from build123d import *

# Parameters (mm, degrees)
F0_W     = 38.1
F0_H     = 76.2
F1_DEPTH = 12.7
F2_R     = 9.525
F3_DEPTH = 38.1
F4_R     = 6.35
F5_DEPTH = 40.386
F6_R     = 2.54
F7_DEPTH = 25.4
F8_R     = 4.445
F9_DEPTH = 7.62


with BuildPart() as f1:
    # F0 (on Front) → F1 (new body)
    with BuildSketch(Plane.XZ):
        Rectangle(F0_W, F0_H)
    extrude(amount=F1_DEPTH)

    # F2 (on face) → F3 (join)
    with BuildSketch(Plane.YZ.offset(19.05)):
        with Locations((-12.7, 0)):
            Circle(F2_R)
    extrude(amount=-F3_DEPTH)

    # F4 (on face) → F5 (cut)
    with BuildSketch(Plane.YZ.offset(19.05)):
        with Locations((-12.7, 0)):
            Circle(F4_R)
    extrude(amount=-F5_DEPTH, mode=Mode.SUBTRACT)

    # F6 (on face) → F7 (cut)
    with BuildSketch(Plane.XZ.offset(12.7)):
        with Locations((-7.62, 25.4)):
            Circle(F6_R)
        with Locations((7.62, 25.4)):
            Circle(F6_R)
        with Locations((-7.62, -25.4)):
            Circle(F6_R)
        with Locations((7.62, -25.4)):
            Circle(F6_R)
    extrude(amount=-F7_DEPTH, mode=Mode.SUBTRACT)

    # F8 (on face) → F9 (cut)
    with BuildSketch(Plane.XZ.offset(12.7)):
        with Locations((-7.62, 25.4)):
            Circle(F8_R)
        with Locations((7.62, 25.4)):
            Circle(F8_R)
        with Locations((-7.62, -25.4)):
            Circle(F8_R)
        with Locations((7.62, -25.4)):
            Circle(F8_R)
    extrude(amount=-F9_DEPTH, mode=Mode.SUBTRACT)


solid = f1.part
Design review of the part built by this model. Coordinates are the model's own, in mm. A direction names the side the tool comes from. Coordinates: 2 decimals unless noted, no trailing zeros. Write each loop counter-clockwise with the first axis right and the second up, starting at its lowest first coordinate (ties: lowest second). Pieces come first, ordered by that corner, then holes. Notation, with made-up numbers: (53.25, -24.75) - (111.25, -24.75) arc R26 ccw to (111.25, -10.75) - close; hole circle Ø9 at (28.25, -13.5). An arc over 180 degrees is marked (long way). Use one line per item in the form item = value.
Q1. For probe 1 along Z at (x, y) = (-7.62, -3.4); probe 2 along Z at (x, y) = (7.62, -8.5) (3 decimals); probe 3 along X at (y, z) = (-4.25, -23.5), list the stretches that pass through material, from the lowest coordinate up.
Taken from the geometry:
probe_1 = -38.1 to -27.94, -22.86 to 22.86, 27.94 to 38.1
probe_2 = -38.1 to -29.845, -20.955 to -4.763, 4.763 to 20.955, 29.845 to 38.1
probe_3 = -19.05 to -9.31, -5.93 to 5.93, 9.31 to 19.05
Q2. Machinability: for faces 4 (the flat face through (0, -12.7, -24)), 5 (the flat face through (10, -5.08, 23)), 6 (the flat face through (0, -6, 38.1)), 7 (the flat face through (0, -12.7, 24)), which of the approach directions +Z, -Z, +X, -X, +Y, -Y give a long, thin tool a straight path to every point of the face, cutting with its end or side? Answer none if there is none.
Taken from the geometry:
face_4 = -Z, +X, -X, -Y
face_5 = -Y
face_6 = +Z, +X, -X, +Y, -Y
face_7 = +Z, +X, -X, -Y
Q3. Consider section D-D (x = -13.5). Write out the cut boundary in (y, z) (3 decimals).
Taken from the geometry:
outline = (-12.7, -38.1) - (0, -38.1) - (0, 38.1) - (-12.7, 38.1) - (-12.7, 9.525) arc R9.525 ccw to (-12.7, -9.525) - close; hole circle Ø12.7 at (-12.7, 0)
Q4. The part is to be moulded in two halves that separate along Y. For faces 1 (the flat face through (-6, -5.08, 23)), 2 (the cylindrical face through (0.267, -6.643, 1.907)), 3 (the cylindrical face through (-6.448, -2.576, -27.653)), say which applies: +Y half, -Y half, draft (parallel to the pull), parting line (faces both ways), or undercut.
Taken from the geometry:
face_1 = -Y half
face_2 = undercut
face_3 = draft
Q5. Consider section B-B (y = -8). Write out the cut boundary in (x, z) (3 decimals), plus the area to 3 significant figures.
Taken from the geometry:
outline = (-19.05, -38.1) - (19.05, -38.1) - (19.05, -4.27) - (-19.05, -4.27) - close; (-19.05, 4.27) - (19.05, 4.27) - (19.05, 38.1) - (-19.05, 38.1) - close; hole circle Ø8.89 at (-7.62, -25.4); hole circle Ø8.89 at (-7.62, 25.4); hole circle Ø8.89 at (7.62, -25.4); hole circle Ø8.89 at (7.62, 25.4)
area = 2,330 mm^2
Q6. Insertion check: pin 1 Ø1 at (x, z) = (-4.5, -20) entering from -Y; pin 2 Ø3 at (x, z) = (7.62, -25.4) entering from +Y; pin 3 Ø8 at (x, z) = (-7.62, -25.4) entering from +Y; pin 4 Ø7 at (x, z) = (-7.62, 25.4) entering from -Y. Each pin has a flat end and moves straight along its axis. Give the tip position at first contact, or say it passes through.
Taken from the geometry:
pin_1 = -12.7
pin_2 = through
pin_3 = 0
pin_4 = -5.08
Q7. Consider section A-A (x = -7.62). Write out the cut boundary in (y, z) (3 decimals), plus the area to 3 significant figures.
Taken from the geometry:
outline = (-12.7, -38.1) - (0, -38.1) - (0, -27.94) - (-5.08, -27.94) - (-5.08, -29.845) - (-12.7, -29.845) - close; (-12.7, -20.955) - (-5.08, -20.955) - (-5.08, -22.86) - (0, -22.86) - (0, 22.86) - (-5.08, 22.86) - (-5.08, 20.955) - (-12.7, 20.955) - (-12.7, 9.525) arc R9.525 ccw to (-12.7, -9.525) - close; (-12.7, 29.845) - (-5.08, 29.845) - (-5.08, 27.94) - (0, 27.94) - (0, 38.1) - (-12.7, 38.1) - close; hole circle Ø12.7 at (-12.7, 0)
area = 796 mm^2
Q8. Consider section C-C (z = 0). Write out the cut boundary in (x, y) (3 decimals), plus the area to 3 significant figures.
Taken from the geometry:
outline = (-19.05, -22.225) - (19.05, -22.225) - (19.05, -19.05) - (-19.05, -19.05) - close; (-19.05, -6.35) - (19.05, -6.35) - (19.05, 0) - (-19.05, 0) - close
area = 363 mm^2
